from build123d import *

# Parameters (mm, degrees)
SKETCH_R     = 2
PAD_DEPTH    = 2
SKETCH001_R  = 19.675731
POCKET_DEPTH = 1


with BuildPart() as part:
    # Sketch → Pad (new body)
    with BuildSketch(Plane.XY):
        with BuildLine():
            ThreePointArc((6.445203, 34.261903), (1.87868, 38.12132), (5.738097, 33.554797))
            Line((5.738097, 33.554797), (9.045739, 30.247154))
            ThreePointArc((9.045739, 30.247154), (5, 20), (9.045739, 9.752846))
            Line((9.045739, 9.752846), (5.738097, 6.445203))
            ThreePointArc((5.738097, 6.445203), (1.87868, 1.87868), (6.445203, 5.738097))
            Line((6.445203, 5.738097), (9.752846, 9.045739))
            ThreePointArc((9.752846, 9.045739), (20, 5), (30.247154, 9.045739))
            Line((33.554797, 5.738097), (30.247154, 9.045739))
            ThreePointArc((33.554797, 5.738097), (38.12132, 1.87868), (34.261903, 6.445203))
            Line((34.261903, 6.445203), (30.954261, 9.752846))
            ThreePointArc((30.954261, 9.752846), (35, 20), (30.954261, 30.247154))
            Line((30.954261, 30.247154), (34.261903, 33.554797))
            ThreePointArc((34.261903, 33.554797), (38.12132, 38.12132), (33.554797, 34.261903))
            Line((33.554797, 34.261903), (30.247154, 30.954261))
            ThreePointArc((30.247154, 30.954261), (20, 35), (9.752846, 30.954261))
            Line((6.445203, 34.261903), (9.752846, 30.954261))
        make_face()
        with Locations((4, 36)):
            Circle(SKETCH_R, mode=Mode.SUBTRACT)
        with Locations((36, 36)):
            Circle(SKETCH_R, mode=Mode.SUBTRACT)
        with Locations((4, 4)):
            Circle(SKETCH_R, mode=Mode.SUBTRACT)
        with Locations((36, 4)):
            Circle(SKETCH_R, mode=Mode.SUBTRACT)
        with BuildLine():
            ThreePointArc((30.246733, 10.460374), (34, 20), (30.246733, 29.539626))
            Line((25.645056, 24.937949), (30.246733, 29.539626))
            ThreePointArc((25.645056, 15.062051), (27.5, 20), (25.645056, 24.937949))
            Line((30.246733, 10.460374), (25.645056, 15.062051))
        make_face(mode=Mode.SUBTRACT)
        with BuildLine():
            ThreePointArc((14.354944, 24.937949), (12.5, 20), (14.354944, 15.062051))
            Line((14.354944, 15.062051), (9.753267, 10.460374))
            ThreePointArc((9.753267, 29.539626), (6, 20), (9.753267, 10.460374))
            Line((9.753267, 29.539626), (14.354944, 24.937949))
        make_face(mode=Mode.SUBTRACT)
        with BuildLine():
            ThreePointArc((24.936129, 15.770978), (26.5, 20), (24.936129, 24.229022))
            Line((22.085604, 21.378497), (24.936129, 24.229022))
            ThreePointArc((22.085604, 18.621503), (22.5, 20), (22.085604, 21.378497))
            Line((22.085604, 18.621503), (24.936129, 15.770978))
        make_face(mode=Mode.SUBTRACT)
        with BuildLine():
            ThreePointArc((17.914396, 21.378497), (17.5, 20), (17.914396, 18.621503))
            Line((17.914396, 18.621503), (15.063871, 15.770978))
            ThreePointArc((15.063871, 24.229022), (13.5, 20), (15.063871, 15.770978))
            Line((15.063871, 24.229022), (17.914396, 21.378497))
        make_face(mode=Mode.SUBTRACT)
        with BuildLine():
            Line((10.460374, 30.246733), (15.062051, 25.645056))
            ThreePointArc((24.937949, 25.645056), (20, 27.5), (15.062051, 25.645056))
            Line((29.539626, 30.246733), (24.937949, 25.645056))
            ThreePointArc((29.539626, 30.246733), (20, 34), (10.460374, 30.246733))
        make_face(mode=Mode.SUBTRACT)
        with BuildLine():
            Line((15.770978, 24.936129), (18.621503, 22.085604))
            ThreePointArc((21.378497, 22.085604), (20, 22.5), (18.621503, 22.085604))
            Line((24.229022, 24.936129), (21.378497, 22.085604))
            ThreePointArc((24.229022, 24.936129), (20, 26.5), (15.770978, 24.936129))
        make_face(mode=Mode.SUBTRACT)
        with BuildLine():
            Line((24.937949, 14.354944), (29.539626, 9.753267))
            ThreePointArc((10.460374, 9.753267), (20, 6), (29.539626, 9.753267))
            Line((10.460374, 9.753267), (15.062051, 14.354944))
            ThreePointArc((15.062051, 14.354944), (20, 12.5), (24.937949, 14.354944))
        make_face(mode=Mode.SUBTRACT)
        with BuildLine():
            Line((24.229022, 15.063871), (21.378497, 17.914396))
            ThreePointArc((18.621503, 17.914396), (20, 17.5), (21.378497, 17.914396))
            Line((15.770978, 15.063871), (18.621503, 17.914396))
            ThreePointArc((15.770978, 15.063871), (20, 13.5), (24.229022, 15.063871))
        make_face(mode=Mode.SUBTRACT)
    extrude(amount=PAD_DEPTH)

    # Sketch001 (on Face54 of Pad) → Pocket (cut)
    with BuildSketch(Plane.XY.offset(2)):
        with Locations((20, 20)):
            Circle(SKETCH001_R)
    extrude(amount=-POCKET_DEPTH, mode=Mode.SUBTRACT)


solid = part.part
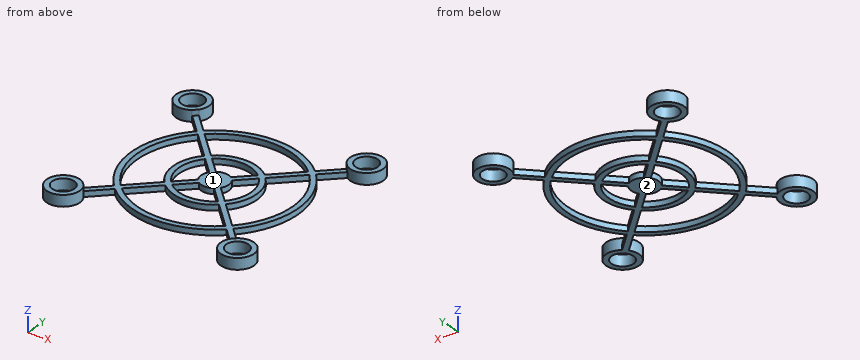
The model under review builds one solid part; all positions refer to its coordinate system, in mm. Face numbers are marked on the shaded views. Give positions to 0.01 mm unless a question says otherwise; leave off trailing zeros. Loops run counter-clockwise (first coordinate to the right, second up) from the corner with the lowest first, then second, coordinate; pieces in that order, holes last. Notation, with made-up numbers: (17, 86) -> (72, 86) arc R27 ccw to (72, 115) -> close; hole circle Ø3 at (-7.5, 89.25). An arc over 180 degrees is marked (long way). Answer as a JSON object with one key per item and string values. Group by question number.
Q1. Take a section at A-A (x = 4). Write out the cut boundary in (y, z).
Q2. Insertion check: pin 1 (10 mm diameter, centred on x = 10.5, y = 15.5, fed in from +Z); pin 2 (4 mm diameter, centred on x = 35, y = 29.5, fed in from -Z). Each pin has a flat end and moves straight along its axis. Give the tip position at first contact, or say it passes through.
Q3. Take a section at C-C (z = 0.35). State how many separate pieces and enclosed holes the cut face has, plus the area to 3 significant figures.
Q4. Draft analysis for pull direction X (two halves, no side actions). For the marked faces 1 and 2, state which applies: pulls with the +X half, pulls with the -X half, needs draft (parallel to the pull), parting line crosses it, or undercut.
Q5. Wall thickness on line 1 along Y through (x, z) = (4, 1); line 2 along Y through (x, z) = (14, 0.15); line 3 along Y through (x, z) = (8, 0.45): over which ranges is each line inside the solid? List them lowest first.
Answer below:
{
 "1": {"outline": "(1, 0) -> (2, 0) -> (2, 2) -> (1, 2) -> close; (6, 0) -> (7, 0) -> (7, 2) -> (6, 2) -> close; (33, 0) -> (34, 0) -> (34, 2) -> (33, 2) -> close; (38, 0) -> (39, 0) -> (39, 2) -> (38, 2) -> close"},
 "2": {"pin 1": "stops at z = 1", "pin 2": "passes through"},
 "3": {"separate pieces": "1", "enclosed holes": "12", "area": "278 mm2"},
 "4": {"face 1": "undercut", "face 2": "needs draft"},
 "5": {"line 1": "y = 1 to 2, 6 to 7, 33 to 34, 38 to 39", "line 2": "y = 6.25 to 7.35, 13.29 to 14.71, 15.5 to 17.5, 22.5 to 24.5, 25.29 to 26.71, 32.65 to 33.75", "line 3": "y = 7.29 to 8.71, 11 to 12.79, 27.21 to 29, 31.29 to 32.71"}
}
